from build123d import *

# Parameters (mm, degrees)
SKETCH3_R           = 2
CUT_EXTRUDE1_DEPTH  = 5
SKETCH4_W           = 12
SKETCH4_H           = 12
BOSS_EXTRUDE1_DEPTH = 5


with BuildPart() as part:
    # Sketch2 → Revolve1 (revolve)
    with BuildSketch(Plane.XY, mode=Mode.PRIVATE) as revolve1_sk:
        Polygon((0, 24.75), (2, 24.75), (8.8, 22.25), (8.8, 7), (0, 7), align=None)
    revolve(revolve1_sk.sketch.rotate(Axis((0, 0, 0), (1, 0, 0)), 90), axis=Axis((0, 0, 0), (1, 0, 0)))

    # Sketch3 → Cut-Extrude1 (cut)
    with BuildSketch(Plane(origin=(8.8, 0, 0), x_dir=(0, 0, -1), z_dir=(1, 0, 0))):
        with Locations((10.606601718, 10.606601718)):
            Circle(SKETCH3_R)
        with Locations((10.606601718, -10.606601718)):
            Circle(SKETCH3_R)
        with Locations((-10.606601718, -10.606601718)):
            Circle(SKETCH3_R)
        with Locations((-10.606601718, 10.606601718)):
            Circle(SKETCH3_R)
    extrude(amount=-CUT_EXTRUDE1_DEPTH, mode=Mode.SUBTRACT)

    # Sketch4 → Boss-Extrude1 (add)
    with BuildSketch(Plane(origin=(8.8, 0, 0), x_dir=(0, 0, -1), z_dir=(1, 0, 0))):
        with Locations((21, 0)):
            Rectangle(SKETCH4_W, SKETCH4_H)
    extrude(amount=-BOSS_EXTRUDE1_DEPTH)


solid = part.part
The model under review builds one solid part; all positions refer to its coordinate system, in mm. A direction names the side the tool comes from. Give positions to 0.01 mm unless a question says otherwise; leave off trailing zeros. Order: outer loops, then holes, each group sorted by start corner. A loop starts at its lowest first (then second) coordinate and runs counter-clockwise, first axis right, second up. Notation, with made-up numbers: M -1.5,47 L 6.5,47 A24 ccw 6.5,71 Z; hole C -36.75,-20.75 d8. An arc over 180 degrees is marked long. One line per question, with ' | ' between items. Start each with the question number.
1) Consider section C-C, the plane y = 0. Give the boundary of the cut face in (x, z).
2) Consider section B-B, the plane x = 4.5. Give the boundary of the cut face in (y, z), then the cut area to 3 significant figures.
3) For faces 4 (the face through (6, 6, -25)), 5 (the face through (6.335, -9.255, 12.081)), 6 (the face through (6, -6, -25)), list the 3-axis set-ups (+Z, -Z, +X, -X, +Y, -Y) from which the entire face can be reached by the end or side of a thin tool; tool diameter is ignored.
4) Clearance check with flat-ended pins moving along their axes: P1, Ø3, axis at y = -10, z = 10, coming from the +X side; P2, Ø3.5, axis at y = 10.61, z = 10.61, coming from the +X side; P3, Ø3, axis at x = 7, z = 2, coming from the -Y side; P4, Ø1, axis at x = 5, z = 18, coming from the +Y side. State where each tip first meets the part, or that it passes through.
5) Wall thickness on L1, parallel to Z at x = 4, y = 10; L2, parallel to Y at x = 0.5, z = 0; L3, parallel to Y at x = 8.5, z = 5: over which ranges is each line inside the solid? List them lowest first. Write a range as from..to.
6) Consider section A-A, the plane z = 0. Give the boundary of the cut face in (x, y), then the cut area to 3 significant figures.
7) Mouldability with a two-part tool opening along Y and no side actions: class faces 1 (the face through (1.01, -16.73, -18.24)), 2 (the face through (6.34, -8.92, -11.68)), 3 (the face through (8.8, 0, -8)) as pulls with the +Y half, pulls with the -Y half, needs draft (parallel to the pull), parting line crosses it, or undercut.
Found:
1) outline: M 0,-24.75 L 2,-24.75 L 3.8,-24.09 L 3.8,-27 L 8.8,-27 L 8.8,-7 L 0,-7 Z; M 0,7 L 8.8,7 L 8.8,22.25 L 2,24.75 L 0,24.75 Z
2) outline: M -6,-27 L 6,-27 L 6,-23.06 A23.83 ccw long -6,-23.06 Z; hole C -10.61,-10.61 d4; hole C -10.61,10.61 d4; hole C 0,0 d14; hole C 10.61,-10.61 d4; hole C 10.61,10.61 d4 | area: 1,620 mm²
3) face 4: -Z, +X, +Y | face 5: +X | face 6: -Z, +X, -Y
4) P1: stops at x = 8.8 | P2: stops at x = 3.8 | P3: stops at y = -23.39 | P4: stops at y = 15.97
5) L1: z = -21.83..-12.51, -8.7..8.7, 12.51..21.83 | L2: y = -24.75..-7, 7..24.75 | L3: y = -21.79..-4.9, 4.9..21.79
6) outline: M 0,-24.75 L 2,-24.75 L 8.8,-22.25 L 8.8,-7 L 0,-7 Z; M 0,7 L 8.8,7 L 8.8,22.25 L 2,24.75 L 0,24.75 Z | area: 295 mm²
7) face 1: parting line crosses it | face 2: undercut | face 3: needs draft
